Geometry: final body of the model. Coordinates: model frame, mm. A direction names the side the tool comes from. Give positions to 0.01 mm unless a question says otherwise; leave off trailing zeros. Write each loop counter-clockwise with the first axis right and the second up, starting at its lowest first coordinate (ties: lowest second). Pieces come first, ordered by that corner, then holes. Notation, with made-up numbers: (71.5, 51.25) - (94.5, 51.25) arc R22 ccw to (94.5, 79.25) - close; hole circle Ø11 at (-11.5, -39.75). An arc over 180 degrees is marked (long way). Use CSV: the item, a comma, the result in double quotes. Start each with the question number.
(1) Reachability of faces 1 (the flat face through (-5, 8, 0)), 2 (the flat face through (0, 16, 15)), 3 (the flat face through (0, 0, 0)) from +Z, -Z, +X, -X, +Y, -Y: full face, straight path, thin tool, end or side. Return the list, or none.
(2) First-contact query: pin 1 Ø13 at (x, z) = (-3.5, 14) entering from -Y. Flat tip, straight axial feed; report the tip coordinate or a pass-through.
(3) Section B-B on z = 13. Output: boundary loops of the cut face in (x, y).
(4) Draft query along Z for faces 4 (the cylindrical face through (-6.5, 1.5, 0)), 5 (the flat face through (0, 10, -2)), 6 (the cylindrical face through (6.386, 18.028, 13.575)), 7 (the flat face through (0, 8, 2)). Return one class per face: released by +Z, released by -Z, zero draft, split by the parting line, or undercut.
(5) Line query: probe 1 along X at (y, z) = (17.8, 13); probe 2 along Z at (x, y) = (5, 18.15); probe 3 along X at (y, z) = (5.75, 0). Output: solid intervals per line, ascending. Write a range as [from, to].
(6) Section D-D on x = -5.5. Output: boundary loops of the cut face in (y, z), and give its area (3 significant figures).
(7) Section C-C on y = 18.75. Output: boundary loops of the cut face in (x, z).
(8) Section A-A on y = 6.5. Output: boundary loops of the cut face in (x, z).
from build123d import *

# Parameters (mm, degrees)
CROQUIS1_W              = 26
CROQUIS1_H              = 4
SALIENTE_EXTRUIR1_DEPTH = 20
CROQUIS2_W              = 26
CROQUIS2_H              = 4
SALIENTE_EXTRUIR2_DEPTH = 26
CROQUIS3_R              = 1.5
CORTAR_EXTRUIR1_DEPTH   = 25
CORTAR_EXTRUIR2_DEPTH   = 25


with BuildPart() as part:
    # Croquis1 → Saliente-Extruir1 (new body)
    with BuildSketch(Plane(origin=(0, 0, 0), x_dir=(1, 0, 0), z_dir=(0, 1, 0))):
        Rectangle(CROQUIS1_W, CROQUIS1_H)
    extrude(amount=SALIENTE_EXTRUIR1_DEPTH)

    # Croquis2 → Saliente-Extruir2 (add)
    with BuildSketch(Plane.XY.offset(2)):
        with Locations((0, 18)):
            Rectangle(CROQUIS2_W, CROQUIS2_H)
    extrude(amount=SALIENTE_EXTRUIR2_DEPTH)

    # Croquis3 → Cortar-Extruir1 (cut)
    with BuildSketch(Plane(origin=(0, 20, 0), x_dir=(1, 0, 0), z_dir=(0, 1, 0))):
        with Locations((-5, -13)):
            Circle(CROQUIS3_R)
        with Locations((5, -13)):
            Circle(CROQUIS3_R)
    extrude(amount=-CORTAR_EXTRUIR1_DEPTH, mode=Mode.SUBTRACT)

    # Croquis4 → Cortar-Extruir2 (cut)
    with BuildSketch(Plane.XY.offset(2)):
        with BuildLine():
            Line((-8, 13), (-8, 3))
            ThreePointArc((-8, 3), (-6.5, 1.5), (-5, 3))
            Line((-5, 3), (-5, 13))
            ThreePointArc((-5, 13), (-6.5, 14.5), (-8, 13))
        make_face()
        with BuildLine():
            Line((5, 13), (5, 3))
            ThreePointArc((5, 3), (6.5, 1.5), (8, 3))
            Line((8, 3), (8, 13))
            ThreePointArc((8, 13), (6.5, 14.5), (5, 13))
        make_face()
    extrude(amount=-CORTAR_EXTRUIR2_DEPTH, mode=Mode.SUBTRACT)


solid = part.part
Check values:
1,face 1,"+Z, -Z"
1,face 2,"+Z, +X, -X, -Y"
1,face 3,"+Z, -Z, +X, -X, -Y"
2,pin 1,"stops at y = 16"
3,outline,"(-13, 16) - (-6.5, 16) - (-6.5, 20) - (-13, 20) - close; (-3.5, 16) - (3.5, 16) - (3.5, 20) - (-3.5, 20) - close; (6.5, 16) - (13, 16) - (13, 20) - (6.5, 20) - close"
4,face 4,"zero draft"
4,face 5,"released by -Z"
4,face 6,"undercut"
4,face 7,"released by +Z"
5,probe 1,"x = [-13, -6.5], [-3.5, 3.5], [6.5, 13]"
5,probe 2,"z = [-2, 11.5], [14.5, 28]"
5,probe 3,"x = [-13, -8], [-5, 5], [8, 13]"
6,outline,"(0, -2) - (1.88, -2) - (1.88, 2) - (0, 2) - close; (14.12, -2) - (20, -2) - (20, 11.59) - (16, 11.59) - (16, 2) - (14.12, 2) - close; (16, 14.41) - (20, 14.41) - (20, 28) - (16, 28) - close"
6,area,"124 mm²"
7,outline,"(-13, -2) - (13, -2) - (13, 28) - (-13, 28) - close; hole circle Ø3 at (-5, 13); hole circle Ø3 at (5, 13)"
8,outline,"(-13, -2) - (-8, -2) - (-8, 2) - (-13, 2) - close; (-5, -2) - (5, -2) - (5, 2) - (-5, 2) - close; (8, -2) - (13, -2) - (13, 2) - (8, 2) - close"
